from build123d import *

# Parameters (mm, degrees)
SKETCH2_W                 = 26.035
SKETCH2_H                 = 15.3416
SKETCH2_R                 = 1.4605
BOSS_EXTRUDE1_DEPTH       = 2.54
SKETCH3_W                 = 26.035
SKETCH3_H                 = 2.54
BOSS_EXTRUDE2_DEPTH       = 38.1
F_4_CLEARANCE_HOLE1_D     = 2.9464
F_4_CLEARANCE_HOLE1_DEPTH = 7.62
F_4_CLEARANCE_HOLE1_TIP   = 0.885187864


with BuildPart() as part:
    # Sketch2 → Boss-Extrude1 (new body)
    with BuildSketch(Plane.XY):
        Rectangle(SKETCH2_W, SKETCH2_H)
        with Locations((-10.4775, 0)):
            Circle(SKETCH2_R, mode=Mode.SUBTRACT)
        with Locations((10.4775, 0)):
            Circle(SKETCH2_R, mode=Mode.SUBTRACT)
    extrude(amount=BOSS_EXTRUDE1_DEPTH)

    # Sketch3 → Boss-Extrude2 (add)
    with BuildSketch(Plane.XY.offset(2.54)):
        with Locations((0, -6.4008)):
            Rectangle(SKETCH3_W, SKETCH3_H)
    extrude(amount=BOSS_EXTRUDE2_DEPTH)

    # #4 Clearance Hole1
    with Locations(Plane(origin=(0, -5.1308, 0), x_dir=(1, 0, 0), z_dir=(0, 1, 0))):
        with Locations((-6.35, -12.065), (6.35, -12.065), (-6.35, -31.115), (6.35, -31.115)):
            Hole(F_4_CLEARANCE_HOLE1_D / 2, depth=F_4_CLEARANCE_HOLE1_DEPTH)
            with Locations((0, 0, -(F_4_CLEARANCE_HOLE1_DEPTH + F_4_CLEARANCE_HOLE1_TIP / 2))):  # 118° drill point
                Cone(0, F_4_CLEARANCE_HOLE1_D / 2, F_4_CLEARANCE_HOLE1_TIP, mode=Mode.SUBTRACT)


solid = part.part
Work out the finished part from the listing and answer in its coordinate system (mm). Coordinates: 2 decimals unless noted, no trailing zeros. Order: outer loops, then holes, each group sorted by start corner. A loop starts at its lowest first (then second) coordinate and runs counter-clockwise, first axis right, second up. Notation, with made-up numbers: (-9, 30) - (20, 30) arc R16 ccw to (20, 49) - close; hole circle Ø1 at (9.5, 78). An arc over 180 degrees is marked (long way). Put each result on its own line as item: value. Start each with the question number.
1) Find section C-C (x = 11.5). Give the vertices of the cut face in (y, z).
2) Find section D-D (z = 16.5). Give the vertices of the cut face in (x, y), plus the area to 3 significant figures.
3) Flat-ended cylindrical pins translate along their axes: pin 1 (10 mm diameter, centred on x = -2, z = 33.5, fed in from +Y); pin 2 (8 mm diameter, centred on x = 3, y = -4, fed in from +Z); pin 3 (4 mm diameter, centred on x = -3.5, y = -2.5, fed in from +Z). Find the tip coordinate at first contact, or state that the pin passes through.
4) For a pull along Y with two mould halves and no side action, classify faces 1 (the cylindrical face through (9.02, 0.06, 1.25)), 2 (the flat face through (0, 1, 2.54)), 3 (the flat face through (0, -5.131, 21)) as released by +Y, released by -Y, zero draft, split by the parting line, or undercut.
5) Find the intervals of material crossed by line 1 (Z direction, x = -6.35, y = -5.9); line 2 (Y direction, x = -10.5, z = 18.5); line 3 (Z direction, x = 6.5, y = 7), in increasing order. Write a range as from..to.
6) Find section B-B (x = 6.35). Give the vertices of the cut face in (y, z).
7) Find section A-A (y = 0). Give the vertices of the cut face in (x, z), plus the area to 3 significant figures.
Results list:
1. outline: (-7.67, 0) - (-1.04, 0) - (-1.04, 2.54) - (-5.13, 2.54) - (-5.13, 40.64) - (-7.67, 40.64) - close; (1.04, 0) - (7.67, 0) - (7.67, 2.54) - (1.04, 2.54) - close
2. outline: (-13.02, -7.67) - (13.02, -7.67) - (13.02, -5.13) - (-13.02, -5.13) - close
2. area: 66.1 mm^2
3. pin 1: stops at y = -5.13
3. pin 2: stops at z = 40.64
3. pin 3: stops at z = 2.54
4. face 1: undercut
4. face 2: zero draft
4. face 3: released by +Y
5. line 1: z = 0..10.59, 13.54..29.64, 32.59..40.64
5. line 2: y = -7.67..-5.13
5. line 3: z = 0..2.54
6. outline: (-7.67, 0) - (7.67, 0) - (7.67, 2.54) - (-5.13, 2.54) - (-5.13, 10.59) - (-7.67, 10.59) - close; (-7.67, 13.54) - (-5.13, 13.54) - (-5.13, 29.64) - (-7.67, 29.64) - close; (-7.67, 32.59) - (-5.13, 32.59) - (-5.13, 40.64) - (-7.67, 40.64) - close
7. outline: (-13.02, 0) - (-11.94, 0) - (-11.94, 2.54) - (-13.02, 2.54) - close; (-9.02, 0) - (9.02, 0) - (9.02, 2.54) - (-9.02, 2.54) - close; (11.94, 0) - (13.02, 0) - (13.02, 2.54) - (11.94, 2.54) - close
7. area: 51.3 mm^2
